from build123d import *

# Parameters (mm, degrees)
SKETCH1_W           = 76.2
SKETCH1_H           = 76.2
BOSS_EXTRUDE1_DEPTH = 25.4
FILLET1_R           = 12.7
SKETCH2_W           = 6.35
SKETCH2_H           = 25.4
SKETCH2_W_2         = 25.4
SKETCH2_H_2         = 6.35
BOSS_EXTRUDE2_DEPTH = 0.00254


with BuildPart() as part:
    # Sketch1 → Boss-Extrude1 (new body)
    with BuildSketch(Plane(origin=(0, 0, 0), x_dir=(1, 0, 0), z_dir=(0, 1, 0))):
        Rectangle(SKETCH1_W, SKETCH1_H)
    extrude(amount=BOSS_EXTRUDE1_DEPTH)

    # Fillet1
    fillet1_edges = [part.edges().sort_by_distance(p)[0] for p in [
        (0, 25.4, 38.1),
        (-38.1, 25.4, 0),
        (0, 25.4, -38.1),
        (-38.1, 0, 0),
        (0, 0, 38.1),
        (38.1, 0, 0),
        (0, 0, -38.1),
        (-38.1, 12.7, -38.1),
        (-38.1, 12.7, 38.1),
        (38.1, 12.7, 38.1),
        (38.1, 12.7, -38.1),
        (38.1, 25.4, 0),
    ]]
    fillet(fillet1_edges, radius=FILLET1_R - 0.0001)  # a hair under: the kernel refuses the full size

    # Sketch2 → Boss-Extrude2 (add)
    with BuildSketch(Plane(origin=(0, 25.4, 0), x_dir=(1, 0, 0), z_dir=(0, 1, 0))):
        Rectangle(SKETCH2_W, SKETCH2_H)
        Rectangle(SKETCH2_W_2, SKETCH2_H_2)
    extrude(amount=BOSS_EXTRUDE2_DEPTH)


solid = part.part
Could you check a few things on this model? Use its own coordinates, in mm. Give positions to 0.01 mm unless a question says otherwise; leave off trailing zeros. Order: outer loops, then holes, each group sorted by start corner. A loop starts at its lowest first (then second) coordinate and runs counter-clockwise, first axis right, second up. Notation, with made-up numbers: (23.5, 50.25) - (31.5, 50.25) arc R28 cw to (31.5, 83.25) - close; hole circle Ø3 at (64.5, 15). An arc over 180 degrees is marked (long way). One line per item, written item: value. Start each with the question number.
1. If I drill on probe 1 along Y at (x, z) = (-2, -17); probe 2 along Y at (x, z) = (-32, 22); probe 3 along X at (y, z) = (4, 3.5), over which ranges is the centre line in solid material (lowest first)?
2. For P1, Ø12, axis at y = 3, z = 24.5, coming from the +X side; P2, Ø1.5, axis at y = 9, z = 9.5, coming from the +X side; P3, Ø2, axis at x = -27, y = 3, coming from the -Z side, each with a flat end and sliding along its axis, tell me the tip position at first contact or that it passes through.
3. Imagine slicing it at C-C on y = 15.75. List the corners of the cut face in (x, z) for me.
Values:
1. probe 1: 0 to 25.4
1. probe 2: 1.85 to 23.55
1. probe 3: -34.65 to 34.65
2. P1: x = 37.55
2. P2: x = 37.75
2. P3: z = -34.53
3. outline: (-37.73, -25.4) arc R12.33 ccw to (-25.4, -37.73) - (25.4, -37.73) arc R12.33 ccw to (37.73, -25.4) - (37.73, 25.4) arc R12.33 ccw to (25.4, 37.73) - (-25.4, 37.73) arc R12.33 ccw to (-37.73, 25.4) - close
